```python
from build123d import *

# Parameters (mm, degrees)
F0_R     = 10
F0_R_2   = 15
F1_DEPTH = 10
F3_DEPTH = 10
F4_W     = 87
F4_H     = 11
F5_DEPTH = 10
F6_W     = 11
F6_H     = 50
F7_DEPTH = 10


with BuildPart() as f1:
    # F0 (on Top) → F1 (new body)
    with BuildSketch(Plane.XY):
        Polygon((150, 110), (-150, 110), (-150, -110), (-69, -110), (150, -110), align=None)
        with Locations((-83.840104, 16.042637)):
            Circle(F0_R, mode=Mode.SUBTRACT)
        with Locations((-18.840104, 1.042637)):
            Circle(F0_R_2, mode=Mode.SUBTRACT)
        with Locations((-18.840104, 41.042637)):
            Circle(F0_R_2, mode=Mode.SUBTRACT)
        with Locations((16.159896, 23.042637)):
            Circle(F0_R_2, mode=Mode.SUBTRACT)
        with Locations((56.159896, 21.042637)):
            Circle(F0_R_2, mode=Mode.SUBTRACT)
        with Locations((96.159896, 19.042637)):
            Circle(F0_R_2, mode=Mode.SUBTRACT)
        with Locations((16.159896, 63.042637)):
            Circle(F0_R_2, mode=Mode.SUBTRACT)
        with Locations((56.159896, 61.042637)):
            Circle(F0_R_2, mode=Mode.SUBTRACT)
        with Locations((96.159896, 59.042637)):
            Circle(F0_R_2, mode=Mode.SUBTRACT)
    extrude(amount=F1_DEPTH)

    # F2 (on face) → F3 (cut)
    with BuildSketch(Plane.XY.offset(10)):
        Polygon((140, 48), (140, 100), (85, 100), (85, 89), (129, 89), (129, 48), align=None)
        Polygon((-85, 100), (-140, 100), (-140, 48), (-129, 48), (-129, 89), (-85, 89), align=None)
        Polygon((-140, -48), (-140, -100), (-85, -100), (-85, -89), (-129, -89), (-129, -48), align=None)
        Polygon((85, -100), (140, -100), (140, -48), (129, -48), (129, -89), (85, -89), align=None)
    extrude(amount=-F3_DEPTH, mode=Mode.SUBTRACT)

    # F4 (on face) → F5 (cut)
    with BuildSketch(Plane.XY.offset(10)):
        with Locations((0, 94.5)):
            Rectangle(F4_W, F4_H)
        with Locations((0, -94.5)):
            Rectangle(F4_W, F4_H)
    extrude(amount=-F5_DEPTH, mode=Mode.SUBTRACT)

    # F6 (on face) → F7 (cut)
    with BuildSketch(Plane.XY.offset(10)):
        with Locations((-134.5, 0)):
            Rectangle(F6_W, F6_H)
        Polygon((140, -25), (140, 0), (140, 25), (129, 25), (129, -25), align=None)
    extrude(amount=-F7_DEPTH, mode=Mode.SUBTRACT)


solid = f1.part
```
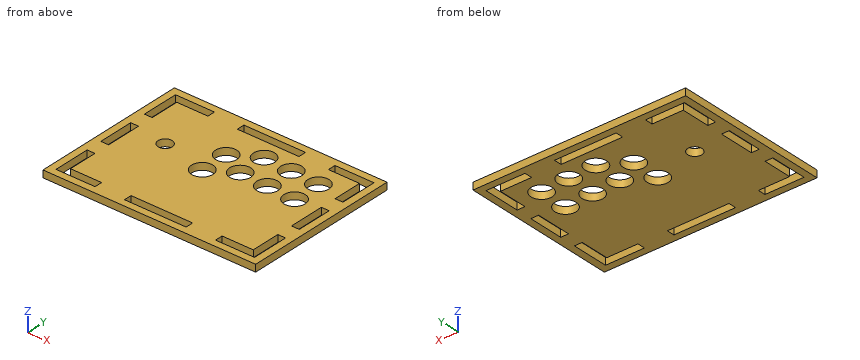
The listing builds one solid part. Answer for the finished solid, in the listing's coordinates (mm). Coordinates: 2 decimals unless noted, no trailing zeros. Write each loop counter-clockwise with the first axis right and the second up, starting at its lowest first coordinate (ties: lowest second). Pieces come first, ordered by that corner, then holes. Notation, with made-up numbers: (11.25, 47.5) - (54.25, 47.5) arc R18 ccw to (54.25, 70.5) - close; hole circle Ø2 at (21.25, 25.25). An arc over 180 degrees is marked (long way). Return JSON: item names as keys, results as strings. Group by question number.
Q1. Find the intervals of material crossed by line 1 along X through (y, z) = (-21, 1.75); line 2 along Y through (x, z) = (-132.5, 1.75); line 3 along Y through (x, z) = (-128, 1.5), in increasing order. Write a range as [from, to].
Q2. A flat-ended cylindrical pin translates along its axis: pin 1 Ø18 at (x, y) = (56.16, 61.04) entering from +Z. Find the tip coordinate at first contact, or state that the pin passes through.
Q3. The part is cut by section C-C on y = 68.5. Write down the section's boundary in (x, z) (3 decimals), and give its area (3 significant figures).
Q4. The part is cut by section D-D on x = -90. Write down the section's boundary in (y, z), and give its area (3 significant figures).
Q5. The part is cut by section B-B on x = 34.5. Write down the section's boundary in (y, z), and give its area (3 significant figures).
Q6. The part is cut by section A-A on y = -94.5. Write down the section's boundary in (x, z), and give its area (3 significant figures).
Evaluation:
{
 "1": {"line 1": "x = [-150, -140], [-129, 129], [140, 150]", "line 2": "y = [-110, -100], [-48, -25], [25, 48], [100, 110]", "line 3": "y = [-110, -100], [-89, 89], [100, 110]"},
 "2": {"pin 1": "passes through"},
 "3": {"outline": "(-150, 0) - (-140, 0) - (-140, 10) - (-150, 10) - close; (-129, 0) - (2.188, 0) - (2.188, 10) - (-129, 10) - close; (30.132, 0) - (43.145, 0) - (43.145, 10) - (30.132, 10) - close; (69.175, 0) - (84.517, 0) - (84.517, 10) - (69.175, 10) - close; (107.803, 0) - (129, 0) - (129, 10) - (107.803, 10) - close; (140, 0) - (150, 0) - (150, 10) - (140, 10) - close", "area": "2,010 mm2"},
 "4": {"outline": "(-110, 0) - (-100, 0) - (-100, 10) - (-110, 10) - close; (-89, 0) - (8.17, 0) - (8.17, 10) - (-89, 10) - close; (23.92, 0) - (89, 0) - (89, 10) - (23.92, 10) - close; (100, 0) - (110, 0) - (110, 10) - (100, 10) - close", "area": "1,820 mm2"},
 "5": {"outline": "(-110, 0) - (-100, 0) - (-100, 10) - (-110, 10) - close; (-89, 0) - (89, 0) - (89, 10) - (-89, 10) - close; (100, 0) - (110, 0) - (110, 10) - (100, 10) - close", "area": "1,980 mm2"},
 "6": {"outline": "(-150, 0) - (-140, 0) - (-140, 10) - (-150, 10) - close; (-85, 0) - (-43.5, 0) - (-43.5, 10) - (-85, 10) - close; (43.5, 0) - (85, 0) - (85, 10) - (43.5, 10) - close; (140, 0) - (150, 0) - (150, 10) - (140, 10) - close", "area": "1,030 mm2"}
}
